from build123d import *

# Parameters (mm, degrees)
SKETCH1_R           = 2.7
BOSS_EXTRUDE1_DEPTH = 3
SKETCH2_R           = 1.696293742
BOSS_EXTRUDE2_DEPTH = 11.6
CUT_EXTRUDE1_DEPTH  = 2


with BuildPart() as part:
    # Sketch1 → Boss-Extrude1 (new body)
    with BuildSketch(Plane(origin=(0, 0, 0), x_dir=(1, 0, 0), z_dir=(0, 1, 0))):
        with Locations((184.714490272, -125.24429514)):
            Circle(SKETCH1_R)
    extrude(amount=-BOSS_EXTRUDE1_DEPTH)

    # Sketch2 → Boss-Extrude2 (add)
    with BuildSketch(Plane.XZ.offset(3)):
        with Locations((184.714490272, 125.24429514)):
            Circle(SKETCH2_R)
    extrude(amount=BOSS_EXTRUDE2_DEPTH)

    # Sketch3 → Cut-Extrude1 (cut)
    with BuildSketch(Plane(origin=(0, 0, 0), x_dir=(1, 0, 0), z_dir=(0, 1, 0))):
        Polygon((184.714490272, -123.800919467), (183.464490272, -124.522607304), (183.464490272, -125.965982977), (184.714490272, -126.687670813), (185.964490272, -125.965982977), (185.964490272, -124.522607304), align=None)
    extrude(amount=-CUT_EXTRUDE1_DEPTH, mode=Mode.SUBTRACT)


solid = part.part
Check sheet for the modelled part. Datum: model origin and axes. Units: mm. A direction names the side the tool comes from. Give positions to 0.01 mm unless a question says otherwise; leave off trailing zeros. Loops run counter-clockwise (first coordinate to the right, second up) from the corner with the lowest first, then second, coordinate; pieces in that order, holes last. Notation, with made-up numbers: M 5,17.5 L 44,17.5 A15 ccw 44,29.5 Z; hole C -26.75,88 d5. An arc over 180 degrees is marked long. Return JSON: item names as keys, results as strings. Group by question number.
1. Cross-section at B-B on y = -1.5. Record the boundary of the cut face in (x, z).
2. Thickness scan on L1, parallel to Y at x = 186.8, z = 123.6; L2, parallel to X at y = -0.25, z = 124; L3, parallel to X at y = -13.5, z = 126.4. Record the ranges inside material, lowest first.
3. Cross-section at C-C on z = 126.45. Record the boundary of the cut face in (x, y), plus the area to 3 significant figures.
4. Mould release check, pull along Z, two halves, no side actions. Record for faces 4 (the cylindrical face through (183.37, -8.72, 124.21)), 5 (the flat face through (184, 0, 124)), 6 (the flat face through (185.35, -0.99, 124.17)): released by +Z, released by -Z, zero draft, split by the parting line, or undercut.
5. Cross-section at A-A on x = 186.2. Record the boundary of the cut face in (y, z), plus the area to 3 significant figures.
6. Tool access check on faces 1 (the flat face through (183, -3, 126)), 2 (the cylindrical face through (182.017, -1.479, 125.126)), 3 (the flat face through (185, -2, 125)). Record the directions out of +Z, -Z, +X, -X, +Y, -Y that give a thin tool (end or side, any length) a straight path to the whole face; none if there is none.
7. Go/stop test with flat-tipped pins: pin 1 (1 mm diameter, centred on x = 186.5, z = 127, fed in from -Y); pin 2 (2 mm diameter, centred on x = 184.5, y = -7.5, fed in from +Z). Record where each tip stops, or that it passes through.
8. Cross-section at D-D on x = 185.4. Record the boundary of the cut face in (y, z), plus the area to 3 significant figures.
Return value:
{
 "1": {"outline": "C 184.71,125.24 d5.4; hole M 183.46,124.52 L 184.71,123.8 L 185.96,124.52 L 185.96,125.97 L 184.71,126.69 L 183.46,125.97 Z"},
 "2": {"L1": "-3 to 0", "L2": "182.32 to 184.37, 185.06 to 187.11", "L3": "183.47 to 185.96"},
 "3": {"outline": "M 182.3,-3 L 183.52,-3 L 183.52,-14.6 L 185.91,-14.6 L 185.91,-3 L 187.13,-3 L 187.13,0 L 185.13,0 L 185.13,-2 L 184.3,-2 L 184.3,0 L 182.3,0 Z", "area": "40.5 mm^2"},
 "4": {"face 4": "split by the parting line", "face 5": "zero draft", "face 6": "undercut"},
 "5": {"outline": "M -14.6,124.43 L -3,124.43 L -3,122.99 L 0,122.99 L 0,127.5 L -3,127.5 L -3,126.06 L -14.6,126.06 Z", "area": "32.5 mm^2"},
 "6": {"face 1": "-Y", "face 2": "+Y, -Y", "face 3": "+Y"},
 "7": {"pin 1": "y = -3", "pin 2": "z = 126.94"},
 "8": {"outline": "M -14.6,123.69 L -3,123.69 L -3,122.63 L 0,122.63 L 0,124.2 L -2,124.2 L -2,126.29 L 0,126.29 L 0,127.86 L -3,127.86 L -3,126.8 L -14.6,126.8 Z", "area": "47.5 mm^2"}
}
